Geometry: final body of the model. Coordinates: model frame, mm. Face numbers are marked on the shaded views. A direction names the side the tool comes from. Coordinates: 2 decimals unless noted, no trailing zeros. Order: outer loops, then holes, each group sorted by start corner. A loop starts at its lowest first (then second) coordinate and runs counter-clockwise, first axis right, second up. Notation, with made-up numbers: M 17.5,89.5 L 28.5,89.5 A21 cw 28.5,99.5 Z; hole C 81.25,-40 d11. An arc over 180 degrees is marked long. Write item = value, one per line. Start each with the question number.
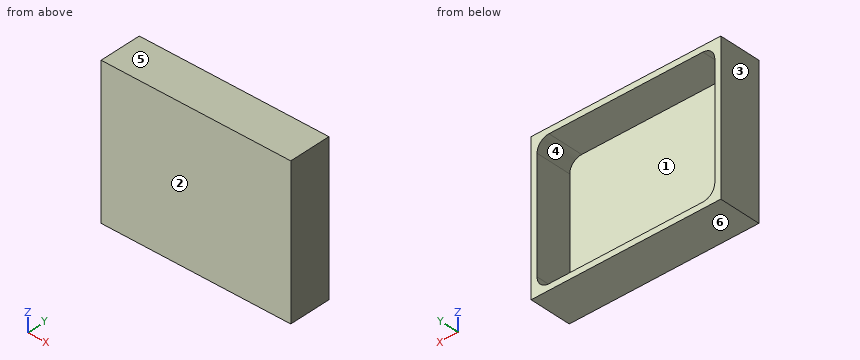
```python
from build123d import *

# Parameters (mm, degrees)
F0_W     = 80.8320604265
F0_H     = 63.012579456
F1_DEPTH = 17.78
F2_T     = -2.54
F3_R     = 5.08


with BuildPart() as f1:
    # F0 (on Front) → F1 (new body)
    with BuildSketch(Plane.XZ):
        with Locations((5.305705592, -7.3265088722)):
            Rectangle(F0_W, F0_H)
    extrude(amount=F1_DEPTH)

    # F2
    f2_openings = [f1.faces().sort_by_distance(p)[0] for p in [
        (5.305706, 0, -7.326509),
    ]]
    offset(amount=F2_T, openings=f2_openings)

    # F3
    f3_edges = [f1.edges().sort_by_distance(p)[0] for p in [
        (-32.570325, -7.62, 21.639781),
        (43.181736, -7.62, 21.639781),
        (43.181736, -7.62, -36.292799),
        (-32.570325, -7.62, -36.292799),
    ]]
    fillet(f3_edges, radius=F3_R)


solid = f1.part
```
Item 1: First-contact query: pin 1 (12 mm diameter, centred on x = 36.5, z = -7, fed in from +Y). Flat tip, straight axial feed; report the tip coordinate or a pass-through.
Item 2: Section query A-A on x = 30. Output: boundary loops of the cut face in (y, z).
Item 3: Section query B-B on y = -2.75. Output: boundary loops of the cut face in (x, z).
Item 4: Draft query along Z for the marked faces 3, 4, 5 and 6. Return one class per face: pulls with the +Z half, pulls with the -Z half, needs draft (parallel to the pull), parting line crosses it, or undercut.
Item 5: Section query C-C on z = -30. Output: boundary loops of the cut face in (x, y).
Item 6: Material intervals for probe 1 along X at (y, z) = (-8.5, 11); probe 2 along Z at (x, y) = (-27, -0.75); probe 3 along Z at (x, y) = (-28.5, -1), sorted ascending. Write a range as [from, to].
Item 7: Reachability of the marked faces 1 and 2 from +Z, -Z, +X, -X, +Y, -Y: full face, straight path, thin tool, end or side. Return the list, or none.
Ans:
q1.pin_1 = -15.24
q2.outline = M -17.78,-38.83 L 0,-38.83 L 0,-36.29 L -15.24,-36.29 L -15.24,21.64 L 0,21.64 L 0,24.18 L -17.78,24.18 Z
q3.outline = M -35.11,-38.83 L 45.72,-38.83 L 45.72,24.18 L -35.11,24.18 Z; hole M -32.57,-31.21 A5.08 ccw -27.49,-36.29 L 38.1,-36.29 A5.08 ccw 43.18,-31.21 L 43.18,16.56 A5.08 ccw 38.1,21.64 L -27.49,21.64 A5.08 ccw -32.57,16.56 Z
q4.face_3 = needs draft
q4.face_4 = undercut
q4.face_5 = pulls with the +Z half
q4.face_6 = pulls with the -Z half
q5.outline = M -35.11,-17.78 L 45.72,-17.78 L 45.72,0 L 43.18,0 L 43.18,-15.24 L -32.57,-15.24 L -32.57,0 L -35.11,0 Z
q6.probe_1 = [-35.11, -32.57], [43.18, 45.72]
q6.probe_2 = [-38.83, -36.29], [21.64, 24.18]
q6.probe_3 = [-38.83, -36.19], [21.54, 24.18]
q7.face_1 = +Y
q7.face_2 = +Z, -Z, +X, -X, -Y
